The model under review builds one solid part; all positions refer to its coordinate system, in mm. Face numbers are marked on the shaded views. Coordinates: 2 decimals unless noted, no trailing zeros. Write each loop counter-clockwise with the first axis right and the second up, starting at its lowest first coordinate (ties: lowest second). Pieces come first, ordered by that corner, then holes. Notation, with made-up numbers: (35.25, 28) - (46.25, 28) arc R29 cw to (46.25, 63) - close; hole circle Ø9 at (3, 42.5). An arc over 180 degrees is marked (long way). Put each result on its own line as item: value.
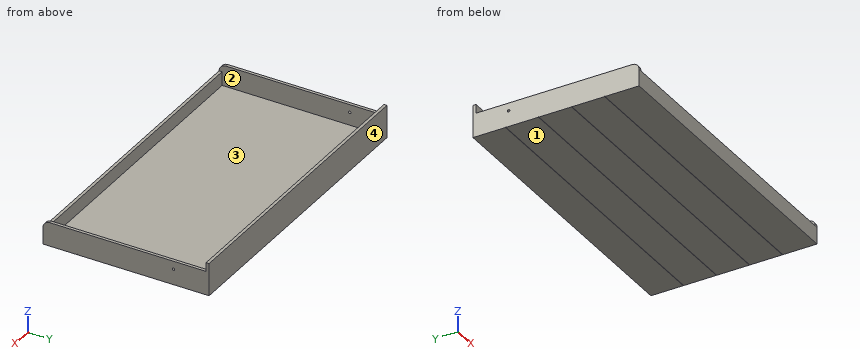
from build123d import *

# Parameters (mm, degrees)
F0_W      = 1930.4
F0_H      = 1066.8
F1_DEPTH  = 19.05
F2_W      = 1930.4
F2_H      = 19.05
F3_DEPTH  = 88.9
F4_W      = 1930.4
F4_H      = 19.05
F5_DEPTH  = 190.5
F7_DEPTH  = 19.05
F9_DEPTH  = 19.05
F10_R     = 7.9375
F11_DEPTH = 1930.401
F12_W     = 3.175
F12_H     = 3.175
F13_DEPTH = 1930.4


with BuildPart() as f1:
    # F0 (on Top) → F1 (new body)
    with BuildSketch(Plane.XY):
        Rectangle(F0_W, F0_H)
    extrude(amount=F1_DEPTH)

    # F2 (on face) → F3 (join)
    with BuildSketch(Plane.XY.offset(19.05)):
        with Locations((0, -523.875)):
            Rectangle(F2_W, F2_H)
    extrude(amount=F3_DEPTH)

    # F4 (on face) → F5 (join)
    with BuildSketch(Plane.XY.offset(19.05)):
        with Locations((0, 523.875)):
            Rectangle(F4_W, F4_H)
    extrude(amount=F5_DEPTH)

    # F6 (on face) → F7 (join)
    with BuildSketch(Plane(origin=(-965.2, 0, 0), x_dir=(0, -1, 0), z_dir=(-1, 0, 0))):
        with BuildLine():
            Line((-533.4, 0), (533.4, 0))
            Line((533.4, 0), (533.4, 107.95))
            ThreePointArc((533.4, 107.95), (520.380896, 139.380896), (488.95, 152.4))
            Line((488.95, 152.4), (-533.4, 152.4))
            Line((-533.4, 152.4), (-533.4, 0))
        make_face()
    extrude(amount=-F7_DEPTH)

    # F8 (on face) → F9 (join)
    with BuildSketch(Plane.YZ.offset(965.2)):
        with BuildLine():
            Line((-533.4, 107.95), (-533.4, 0))
            Line((-533.4, 0), (533.4, 0))
            Line((533.4, 0), (533.4, 152.4))
            Line((533.4, 152.4), (-488.95, 152.4))
            ThreePointArc((-488.95, 152.4), (-520.380896, 139.380896), (-533.4, 107.95))
        make_face()
    extrude(amount=-F9_DEPTH)

    # F10 (on face) → F11 (cut, through all)
    with BuildSketch(Plane(origin=(-965.2, 0, 0), x_dir=(0, -1, 0), z_dir=(-1, 0, 0))):
        with Locations((-304.8, 101.6)):
            Circle(F10_R)
    extrude(amount=-F11_DEPTH, mode=Mode.SUBTRACT)

    # F12 (on face) → F13 (cut, through all)
    with BuildSketch(Plane(origin=(-965.2, 0, 0), x_dir=(0, -1, 0), z_dir=(-1, 0, 0))):
        with Locations((-323.5325, 1.5875)):
            Rectangle(F12_W, F12_H)
        with Locations((-111.4425, 1.5875)):
            Rectangle(F12_W, F12_H)
        with Locations((100.6475, 1.5875)):
            Rectangle(F12_W, F12_H)
        with Locations((312.7375, 1.5875)):
            Rectangle(F12_W, F12_H)
    extrude(amount=-F13_DEPTH, mode=Mode.SUBTRACT)


solid = f1.part
1. The part is to be moulded in two halves that separate along Y. For the marked faces 1, 2, 3 and 4, say which applies: +Y half, -Y half, draft (parallel to the pull), parting line (faces both ways), or undercut.
Determined:
face 1: draft
face 2: undercut
face 3: undercut
face 4: +Y half
2. To check wall thickness, follow probe 1 along Z at (x, y) = (957.25, 304.8); probe 2 along X at (y, z) = (-431.5, 93); probe 3 along Y at (x, z) = (-38.5, 55.5). State the ranges of each line that lie inside material, in increasing order.
Determined:
probe 1: z = 0 to 93.66, 109.54 to 152.4
probe 2: x = -965.2 to -946.15, 946.15 to 965.2
probe 3: y = -533.4 to -514.35, 514.35 to 533.4
3. Consider section A-A on y = 145.5. State the section outline as (x, z) points, plus the area to 3 significant figures.
Determined:
outline: (-965.2, 0) - (965.2, 0) - (965.2, 152.4) - (946.15, 152.4) - (946.15, 19.05) - (-946.15, 19.05) - (-946.15, 152.4) - (-965.2, 152.4) - close
area: 41,900 mm^2
4. Consider section C-C on x = -789. State the section outline as (y, z) points (3 decimals).
Determined:
outline: (-533.4, 0) - (-314.325, 0) - (-314.325, 3.175) - (-311.15, 3.175) - (-311.15, 0) - (-102.235, 0) - (-102.235, 3.175) - (-99.06, 3.175) - (-99.06, 0) - (109.855, 0) - (109.855, 3.175) - (113.03, 3.175) - (113.03, 0) - (321.945, 0) - (321.945, 3.175) - (325.12, 3.175) - (325.12, 0) - (533.4, 0) - (533.4, 209.55) - (514.35, 209.55) - (514.35, 19.05) - (-514.35, 19.05) - (-514.35, 107.95) - (-533.4, 107.95) - close
5. Consider section B-B on z = 44. State the section outline as (x, y) points, plus the area to 3 significant figures.
Determined:
outline: (-965.2, -533.4) - (965.2, -533.4) - (965.2, 533.4) - (-965.2, 533.4) - close; hole (-946.15, -514.35) - (946.15, -514.35) - (946.15, 514.35) - (-946.15, 514.35) - close
area: 113,000 mm^2
6. Consider section D-D on z = 128. State the section outline as (x, y) points.
Determined:
outline: (-965.2, -528.62) - (-946.15, -528.62) - (-946.15, 514.35) - (946.15, 514.35) - (946.15, -528.62) - (965.2, -528.62) - (965.2, 533.4) - (-965.2, 533.4) - close
7. For pin 1 Ø1 at (x, y) = (-433, -313) entering from -Z (3 decimals); pin 2 Ø4 at (x, y) = (377.5, -26.5) entering from +Z; pin 3 Ø20.5 at (y, z) = (304.8, 101.6) entering from -X; pin 4 Ø21 at (x, y) = (-956.5, 142.5) entering from +Z, all flat-tipped, find the tip position at first contact; note any pin that passes through.
Determined:
pin 1: stops at z = 3.175
pin 2: stops at z = 19.05
pin 3: stops at x = -965.2
pin 4: stops at z = 152.4
